For this review, take the finished solid that the model builds, in its own axes (mm). Face numbers are marked on the shaded views. Round coordinates to 2 decimals unless told otherwise and drop trailing zeros. Order: outer loops, then holes, each group sorted by start corner. A loop starts at its lowest first (then second) coordinate and runs counter-clockwise, first axis right, second up. Notation, with made-up numbers: M -16.5,7.25 L 34.5,7.25 A23 ccw 34.5,42.25 Z; hole C 64.25,6.25 d4. An arc over 180 degrees is marked long. Use a Markdown table: item, result.
Autodesk Inventor part; units mm, degrees
ref_plane "YZ Plane" through (0, 0, 0) normal (1, 0, 0) x (0, 1, 0)
ref_plane "XZ Plane" through (0, 0, 0) normal (0, 1, 0) x (-1, 0, 0)
ref_plane "XY Plane" through (0, 0, 0) normal (0, 0, 1) x (1, 0, 0)
sketch "Skizze1" plane through (0, 0, 0) normal (0, 0, 1) x (1, 0, 0)
  line L0 (0, 2.8868) -> (2.5, 1.4434)
  line L1 (2.5, 1.4434) -> (2.5, -1.4434)
  line L2 (2.5, -1.4434) -> (0, -2.8868)
  line L3 (0, -2.8868) -> (-2.5, -1.4434)
  line L4 (-2.5, -1.4434) -> (-2.5, 1.4434)
  line L5 (-2.5, 1.4434) -> (0, 2.8868)
  circle A0 centre (0, 0) radius 1.5
  dimension "d0" = 5
  dimension "d1" = 3
extrude "Extrusion1" add sketch "Skizze1" along normal blind 5
chamfer "Fase1" distance 0.3 angle 45 13 edges at (1.25, -2.1651, 5) (-1.25, -2.1651, 5) (2.5, 0, 5) (1.25, 2.1651, 5) (-1.25, 2.1651, 5) (1.25, -2.1651, 0) (2.5, 0, 0) (-1.25, -2.1651, 0) (1.25, 2.1651, 0) (-1.25, 2.1651, 0) (-2.5, 0, 0) (-1.5, 0, 5) (-1.5, 0, 0)
thread "Gewinde1"
properties part number "Distanzhuelse_M3x5mm" material "Nickel-Kupfer-Legierung 400"
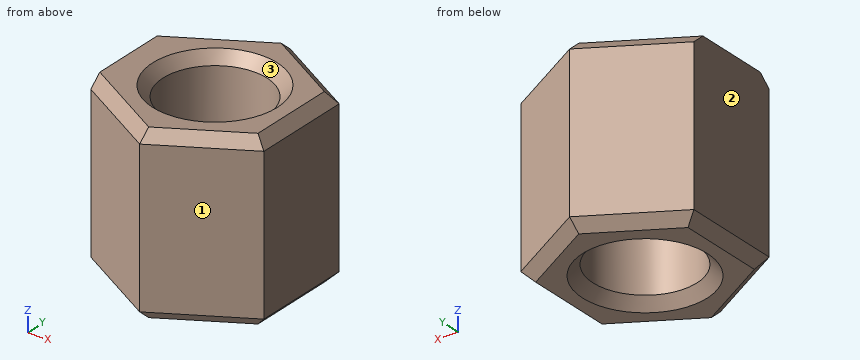
Q1. Add section A-A (y = 0). Write out the cut boundary in (x, z).
Determined:
| item | result |
|---|---|
| outline | M -2.5,0.3 L -2.2,0 L -1.8,0 L -1.5,0.3 L -1.5,4.7 L -1.8,5 L -2.5,5 Z; M 1.5,0.3 L 1.8,0 L 2.2,0 L 2.5,0.3 L 2.5,4.7 L 2.2,5 L 1.8,5 L 1.5,4.7 Z |
Q2. Draft analysis for pull direction Y (two halves, no side actions). For the marked faces 1, 2 and 3, state which applies: pulls with the +Y half, pulls with the -Y half, needs draft (parallel to the pull), parting line crosses it, or undercut.
Determined:
| item | result |
|---|---|
| face 1 | pulls with the -Y half |
| face 2 | needs draft |
| face 3 | undercut |
Q3. Add section D-D (y = 2.4). Write out the cut boundary in (x, z).
Determined:
| item | result |
|---|---|
| outline | M -0.84,0.3 L -0.24,0 L 0.24,0 L 0.84,0.3 L 0.84,4.7 L 0.24,5 L -0.24,5 L -0.84,4.7 Z |
Q4. Wall thickness on line 1 along X through (y, z) = (-0.4, 4.25); line 2 along Y through (x, z) = (0.15, 4.5); line 3 along Y through (x, z) = (-0.9, 1.45): over which ranges is each line inside the solid? List them lowest first. Write a range as [from, to].
Determined:
| item | result |
|---|---|
| line 1 | x = [-2.5, -1.45], [1.45, 2.5] |
| line 2 | y = [-2.8, -1.49], [1.49, 2.8] |
| line 3 | y = [-2.37, -1.2], [1.2, 2.37] |
Q5. Add section C-C (x = -2.1). Write out the cut boundary in (y, z).
Determined:
| item | result |
|---|---|
| outline | M -1.67,0.3 L -1.33,0 L 1.33,0 L 1.67,0.3 L 1.67,4.7 L 1.33,5 L -1.33,5 L -1.67,4.7 Z |
Q6. Add section B-B (z = 3.3). Write out the cut boundary in (x, y), then the cut area to 3 significant figures.
Determined:
| item | result |
|---|---|
| outline | M -2.5,-1.44 L 0,-2.89 L 2.5,-1.44 L 2.5,1.44 L 0,2.89 L -2.5,1.44 Z; hole C 0,0 d3 |
| area | 14.6 mm^2 |
